Check sheet for the modelled part. Datum: model origin and axes. Units: mm. Face numbers are marked on the shaded views. A direction names the side the tool comes from. Coordinates: 2 decimals unless noted, no trailing zeros. Loops run counter-clockwise (first coordinate to the right, second up) from the corner with the lowest first, then second, coordinate; pieces in that order, holes last. Notation, with made-up numbers: (-18, -7) -> (39, -7) arc R7 ccw to (39, 5) -> close; hole circle Ø10 at (-26, 70.25). An arc over 180 degrees is marked (long way). Use one line per item in the form item = value.
from build123d import *

# Parameters (mm, degrees)
F0_W     = 14.2875
F0_H     = 13.49375
F1_DEPTH = 1.5875
F3_DEPTH = 3.175
F4_R     = 0.79375


with BuildPart() as f1:
    # F0 (on Top) → F1 (new body)
    with BuildSketch(Plane.XY):
        Rectangle(F0_W, F0_H)
        with BuildLine():
            ThreePointArc((4.7625, -2.778125), (4.297532, -3.900657), (3.175, -4.365625))
            Line((3.175, -4.365625), (-3.175, -4.365625))
            ThreePointArc((-3.175, -4.365625), (-4.297532, -3.900657), (-4.7625, -2.778125))
            Line((-4.7625, -2.778125), (-4.7625, 2.778125))
            ThreePointArc((-4.7625, 2.778125), (-4.297532, 3.900657), (-3.175, 4.365625))
            Line((-3.175, 4.365625), (3.175, 4.365625))
            ThreePointArc((3.175, 4.365625), (4.297532, 3.900657), (4.7625, 2.778125))
            Line((4.7625, 2.778125), (4.7625, -2.778125))
        make_face(mode=Mode.SUBTRACT)
        with BuildLine():
            Line((-3.175, -4.365625), (3.175, -4.365625))
            ThreePointArc((3.175, -4.365625), (4.297532, -3.900657), (4.7625, -2.778125))
            Line((4.7625, -2.778125), (4.7625, 2.778125))
            ThreePointArc((4.7625, 2.778125), (4.297532, 3.900657), (3.175, 4.365625))
            Line((3.175, 4.365625), (-3.175, 4.365625))
            ThreePointArc((-3.175, 4.365625), (-4.297532, 3.900657), (-4.7625, 2.778125))
            Line((-4.7625, 2.778125), (-4.7625, -2.778125))
            ThreePointArc((-4.7625, -2.778125), (-4.297532, -3.900657), (-3.175, -4.365625))
        make_face()
    extrude(amount=F1_DEPTH)

    # F2 (on face) → F3 (join)
    with BuildSketch(Plane.XY.offset(1.5875)):
        with BuildLine():
            ThreePointArc((4.7625, 2.778125), (4.297532, 3.900657), (3.175, 4.365625))
            Line((3.175, 4.365625), (-3.175, 4.365625))
            ThreePointArc((-3.175, 4.365625), (-4.297532, 3.900657), (-4.7625, 2.778125))
            Line((-4.7625, 2.778125), (-4.7625, -2.778125))
            ThreePointArc((-4.7625, -2.778125), (-4.297532, -3.900657), (-3.175, -4.365625))
            Line((-3.175, -4.365625), (3.175, -4.365625))
            ThreePointArc((3.175, -4.365625), (4.297532, -3.900657), (4.7625, -2.778125))
            Line((4.7625, -2.778125), (4.7625, 2.778125))
        make_face()
    extrude(amount=F3_DEPTH)

    # F4
    f4_edges = [f1.edges().sort_by_distance(p)[0] for p in [
        (4.7625, 0, 4.7625),
    ]]
    fillet(f4_edges, radius=F4_R)


solid = f1.part
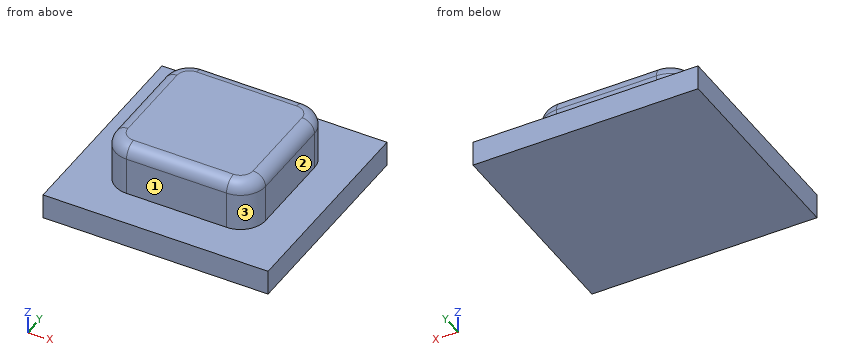
(1) Section check A-A, the plane y = -1.5. Record the boundary of the cut face in (x, z).
Established:
outline = (-7.14, 0) -> (7.14, 0) -> (7.14, 1.59) -> (4.76, 1.59) -> (4.76, 3.97) arc R0.79 ccw to (3.97, 4.76) -> (-3.97, 4.76) arc R0.79 ccw to (-4.76, 3.97) -> (-4.76, 1.59) -> (-7.14, 1.59) -> close
(2) Go/stop test with flat-tipped pins: P1, Ø1.2, axis at x = -0.5, z = 2.5, coming from the -Y side; P2, Ø1, axis at y = -4, z = 2.5, coming from the -X side; P3, Ø1.2, axis at y = 0, z = 3, coming from the +X side. Record where each tip stops, or that it passes through.
Established:
P1 = -4.37
P2 = -4.59
P3 = 4.76
(3) Section check D-D, the plane x = 6. Record the boundary of the cut face in (y, z).
Established:
outline = (-6.75, 0) -> (6.75, 0) -> (6.75, 1.59) -> (-6.75, 1.59) -> close
(4) Section check C-C, the plane x = 2. Record the boundary of the cut face in (y, z).
Established:
outline = (-6.75, 0) -> (6.75, 0) -> (6.75, 1.59) -> (4.37, 1.59) -> (4.37, 3.97) arc R0.79 ccw to (3.57, 4.76) -> (-3.57, 4.76) arc R0.79 ccw to (-4.37, 3.97) -> (-4.37, 1.59) -> (-6.75, 1.59) -> close
(5) Tool access check on the marked faces 1, 2 and 3. Record the directions out of +Z, -Z, +X, -X, +Y, -Y that give a thin tool (end or side, any length) a straight path to the whole face; none if there is none.
Established:
face_1 = +Z, +X, -X, -Y
face_2 = +Z, +X, +Y, -Y
face_3 = +Z, +X, -Y
(6) Scan lines: line 1 along X through (y, z) = (1, 3.55); line 2 along Z through (x, y) = (-5, -2); line 3 along Y through (x, z) = (-1.5, 4.2). Record each from-to range of solid material in increasing order.
Established:
line_1 = -4.76 to 4.76
line_2 = 0 to 1.59
line_3 = -4.33 to 4.33
(7) Section check B-B, the plane z = 2.25. Record the boundary of the cut face in (x, y) (1 decimal).
Established:
outline = (-4.8, -2.8) arc R1.6 ccw to (-3.2, -4.4) -> (3.2, -4.4) arc R1.6 ccw to (4.8, -2.8) -> (4.8, 2.8) arc R1.6 ccw to (3.2, 4.4) -> (-3.2, 4.4) arc R1.6 ccw to (-4.8, 2.8) -> close
